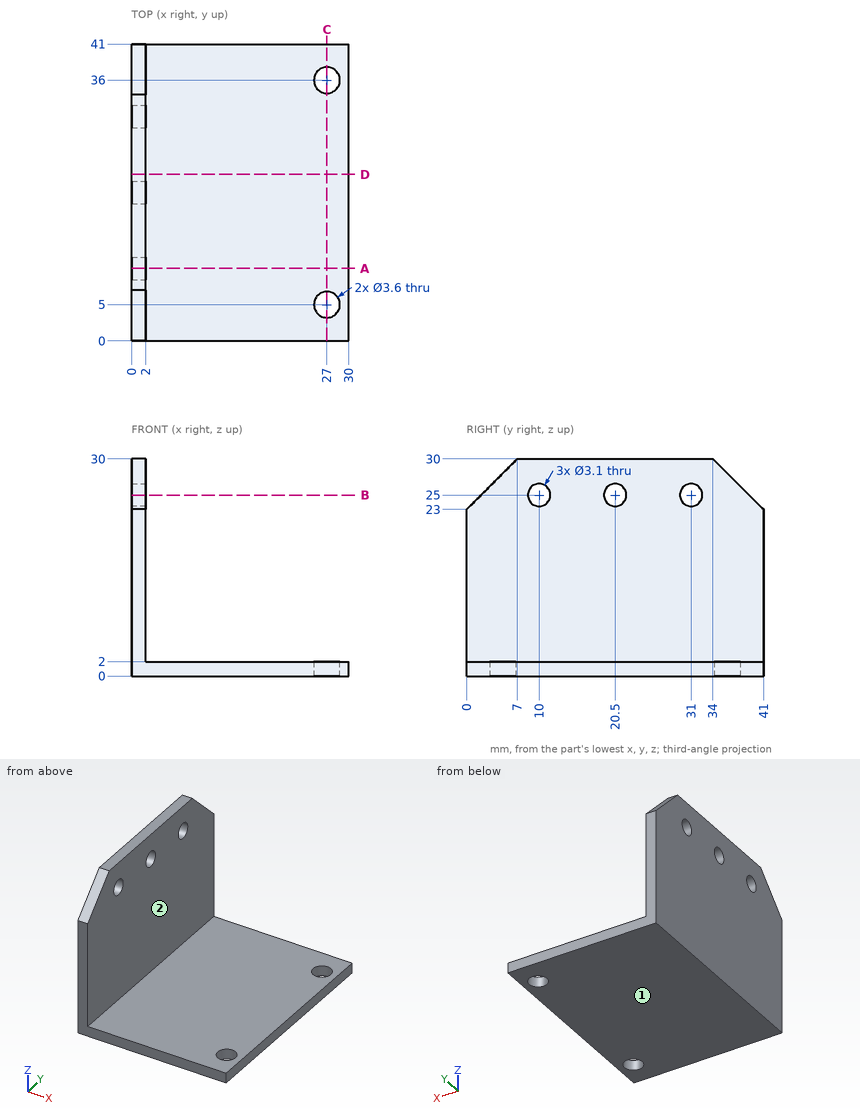
Input: dimensioned drawing with shaded views. Units: mm. Origin: part minimum x, y, z. A direction names the side the tool comes from. Give positions to 0.01 mm unless a question says otherwise; leave off trailing zeros. Write each loop counter-clockwise with the first axis right and the second up, starting at its lowest first coordinate (ties: lowest second). Pieces come first, ordered by that corner, then holes. Notation, with made-up numbers: (10, -14.75) -> (48, -14.75) arc R18 cw to (48, -4.75) -> close; hole circle Ø1 at (16.5, -0.75). An arc over 180 degrees is marked (long way). Return JSON: item names as keys, results as strings. Group by question number.
1. Access query for the marked faces 1 and 2. Directions: +Z, -Z, +X, -X, +Y, -Y. A direction counts if a zero-diameter tool reaches every point of the face in a straight line with its end or side. Return the directions, or none.
2. Section C-C, the plane x = 27. Output: boundary loops of the cut face in (y, z).
3. Section D-D, the plane y = 23. Output: boundary loops of the cut face in (x, z).
4. Pin query (flat end, axial travel): pin 1 Ø5 at (y, z) = (20.5, 25) entering from -X; pin 2 Ø14 at (x, y) = (20.5, 10.5) entering from +Z; pin 3 Ø3 at (y, z) = (14, 10) entering from +X. Return the tip coordinate at first contact, or that it passes through.
5. Material intervals for line 1 (Y direction, x = 0.5, z = 25); line 2 (X direction, y = 35, z = 7), sorted ascending. Write a range as from..to.
6. Section B-B, the plane z = 25. Output: boundary loops of the cut face in (x, y).
7. Section A-A, the plane y = 10. Output: boundary loops of the cut face in (x, z), then the cut area to 3 significant figures.
Determined:
{
 "1": {"face 1": "-Z, +X, -X, +Y, -Y", "face 2": "+Z, +X, +Y, -Y"},
 "2": {"outline": "(0, 0) -> (3.2, 0) -> (3.2, 2) -> (0, 2) -> close; (6.8, 0) -> (34.2, 0) -> (34.2, 2) -> (6.8, 2) -> close; (37.8, 0) -> (41, 0) -> (41, 2) -> (37.8, 2) -> close"},
 "3": {"outline": "(0, 0) -> (30, 0) -> (30, 2) -> (2, 2) -> (2, 30) -> (0, 30) -> close"},
 "4": {"pin 1": "stops at x = 0", "pin 2": "stops at z = 2", "pin 3": "stops at x = 2"},
 "5": {"line 1": "y = 2..8.45, 11.55..18.95, 22.05..29.45, 32.55..39", "line 2": "x = 0..2"},
 "6": {"outline": "(0, 2) -> (2, 2) -> (2, 8.45) -> (0, 8.45) -> close; (0, 11.55) -> (2, 11.55) -> (2, 18.95) -> (0, 18.95) -> close; (0, 22.05) -> (2, 22.05) -> (2, 29.45) -> (0, 29.45) -> close; (0, 32.55) -> (2, 32.55) -> (2, 39) -> (0, 39) -> close"},
 "7": {"outline": "(0, 0) -> (30, 0) -> (30, 2) -> (2, 2) -> (2, 23.45) -> (0, 23.45) -> close; (0, 26.55) -> (2, 26.55) -> (2, 30) -> (0, 30) -> close", "area": "110 mm2"}
}
